Geometry check sheet. Reference: drawing and pictorial views, mm from the part's lowest x, y, z. A direction names the side the tool comes from. Give positions to 0.01 mm unless a question says otherwise; leave off trailing zeros. Write each loop counter-clockwise with the first axis right and the second up, starting at its lowest first coordinate (ties: lowest second). Pieces come first, ordered by that corner, then holes. Notation, with made-up numbers: (13, -12) -> (34, -12) arc R20 ccw to (34, 25) -> close; hole circle Ø11 at (-4.5, 3.25). An arc over 180 degrees is marked (long way). Use a Markdown table: item, result. Add a question column.
1. Cross-section at B-B (z = 30). Enter the section's corners in (x, y), then the cut area to 3 significant figures.
2. Set-up check for the marked faces 4 and 5: record each of +Z, -Z, +X, -X, +Y, -Y from which the full face is reachable in a straight line by a thin tool's end or side.
3. Scan lines: probe 1 along Z at (x, y) = (46, 1.5); probe 2 along X at (y, z) = (4.5, 31.5); probe 3 along Y at (x, z) = (23, 35.5). Record each from-to range of solid material in increasing order. Write a range as [from, to].
4. Cross-section at A-A (y = 9). Enter the section's corners in (x, z).
5. Gauge pin test, flat ends, axial feed: P1, Ø2, axis at y = 8.5, z = 16, coming from the -X side; P2, Ø4, axis at x = 24, z = 28, coming from the +Y side. Record the tip position at first contact, or that the pin passes through.
6. Cross-section at C-C (x = 6). Enter the section's corners in (y, z).
7. Release check for a two-part mould opening along X. For the marked faces 1, 2 and 3 record: released by +X, released by -X, zero draft, split by the parting line, or undercut.
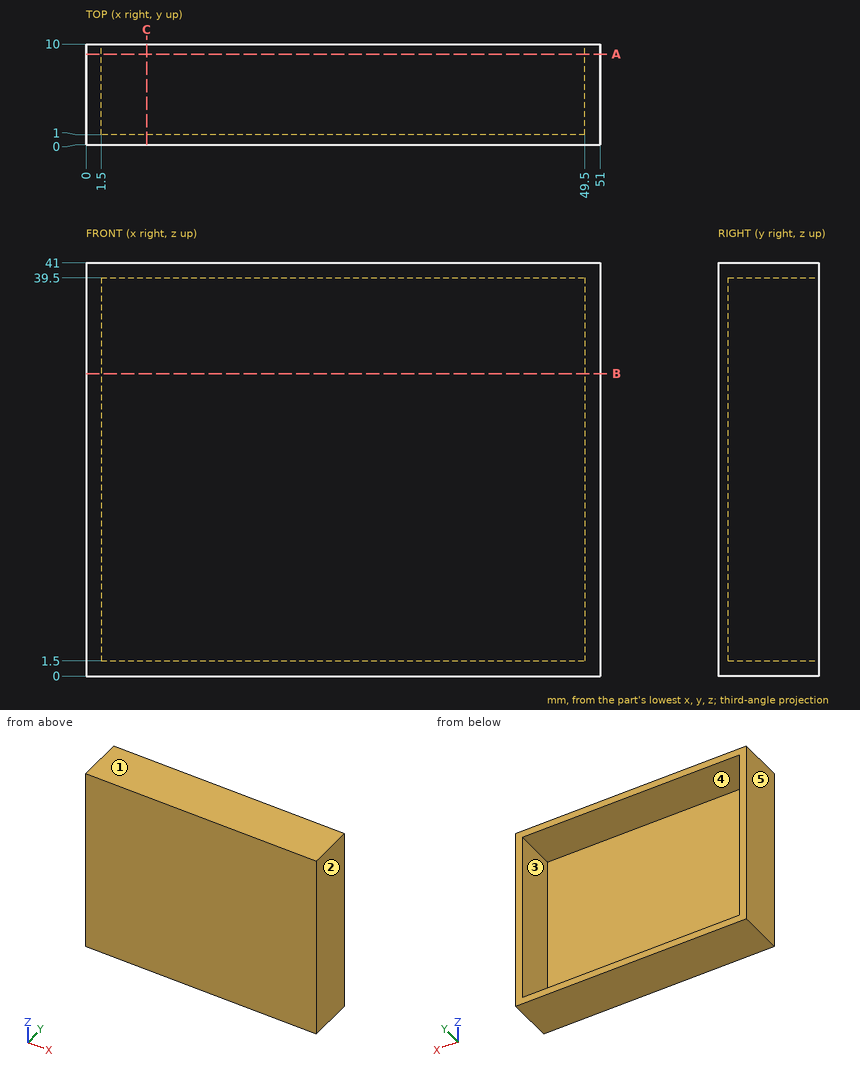
Worked answers:
| question | item | result |
|---|---|---|
| 1 | outline | (0, 0) -> (51, 0) -> (51, 10) -> (49.5, 10) -> (49.5, 1) -> (1.5, 1) -> (1.5, 10) -> (0, 10) -> close |
| 1 | area | 78.0 mm² |
| 2 | face 4 | +Y |
| 2 | face 5 | +Z, -Z, -X, +Y, -Y |
| 3 | probe 1 | z = [0, 1.5], [39.5, 41] |
| 3 | probe 2 | x = [0, 1.5], [49.5, 51] |
| 3 | probe 3 | y = [0, 1] |
| 4 | outline | (0, 0) -> (51, 0) -> (51, 41) -> (0, 41) -> close; hole (1.5, 1.5) -> (49.5, 1.5) -> (49.5, 39.5) -> (1.5, 39.5) -> close |
| 5 | P1 | stops at x = 0 |
| 5 | P2 | stops at y = 1 |
| 6 | outline | (0, 0) -> (10, 0) -> (10, 1.5) -> (1, 1.5) -> (1, 39.5) -> (10, 39.5) -> (10, 41) -> (0, 41) -> close |
| 7 | face 1 | zero draft |
| 7 | face 2 | released by +X |
| 7 | face 3 | undercut |
